The listing builds one solid part. Answer for the finished solid, in the listing's coordinates (mm). Give positions to 0.01 mm unless a question says otherwise; leave off trailing zeros. Write each loop counter-clockwise with the first axis right and the second up, starting at its lowest first coordinate (ties: lowest second). Pieces come first, ordered by that corner, then holes. Notation, with made-up numbers: (43.5, 58.25) - (74.5, 58.25) arc R20 cw to (74.5, 90.25) - close; hole circle Ø1 at (-12, 5.25). An arc over 180 degrees is marked (long way). Answer as CSV lines item,"result". Start each with the question number.
(1) Find section A-A (y = 77.5). Write down the section's boundary in (x, z), then the cut area to 4 significant figures.
(2) Find section D-D (y = 56.5). Write down the section's boundary in (x, z), then the cut area to 3 significant figures.
(3) Straight lines are drawn through the part: probe 1 along Y at (x, z) = (21.25, 6.75); probe 2 along Y at (x, z) = (16.5, 0.5); probe 3 along X at (y, z) = (34, 0.75). For each, find the intervals that lie inside material, in ascending order.
(4) Each of these flat-tipped pins is pushed along its axis until it touches: pin 1 Ø1.5 at (x, z) = (29.5, 6.5) entering from +Y; pin 2 Ø5 at (y, z) = (29, 8.5) entering from -X; pin 3 Ø7.5 at (x, y) = (21.25, 77.5) entering from -Z; pin 4 Ø5 at (x, z) = (124.5, 4.5) entering from +Y. Where does it stop, or does it pass through?
(5) For a pull along Y with two mould halves and no side action, classify faces 1 (the face through (20.436, 83.697, 4.93)), 2 (the face through (82, -1.25, 5)), 3 (the face through (74, 49, 0)) as pulls with the +Y half, pulls with the -Y half, needs draft (parallel to the pull), parting line crosses it, or undercut.
(6) Find section B-B (z = 2.25). Write down the section's boundary in (x, y), then the cut area to 3 significant figures.
(7) Find section C-C (x = 22). Write down the section's boundary in (y, z).
from build123d import *

# Parameters (mm, degrees)
F0_R        = 6.25
F1_DEPTH    = 10
F2_T1_DEPTH = 18.1439634323
F2_T3_DEPTH = 61.4336597593
F3_R        = 10


# Not quite as in the source:
# - a fillet or chamfer that OpenCascade refuses, or shapes differently, is made with other operations: its cross-section is extruded or revolved along the edge and cut away or added
# - two fillets or chamfers of one size are made in one step


with BuildPart() as f1:
    # F0 (on Top) → F1 (new body)
    with BuildSketch(Plane.XY):
        Polygon((0, 73.75), (15, -1.25), (150, -1.25), (150, 68.75), (30, 98.75), (0, 98.75), align=None)
        with Locations((21.25, 77.5)):
            Circle(F0_R, mode=Mode.SUBTRACT)
    extrude(amount=F1_DEPTH)

    # F2: chamfer of 10 on 2 edges, made by hand

    # F2_s2 → F2_t1 (cut)
    with BuildSketch(Plane.XY.offset(-4.0719817161)):
        Polygon((31.1942999942, 98.4514250015), (28.7689437438, 98.75), (30, 98.75), align=None)
    extrude(amount=F2_T1_DEPTH, mode=Mode.SUBTRACT)

    # F2_s4 → F2_t3 (cut)
    with BuildSketch(Plane.XY.offset(-25.7168298797)):
        Polygon((10, 98.75), (0, 88.75), (0, 98.75), align=None)
    extrude(amount=F2_T3_DEPTH, mode=Mode.SUBTRACT)

    # F3
    f3_edges = [f1.edges().sort_by_distance(p)[0] for p in [
        (0, 88.75, 5),
        (10, 98.75, 5),
        (28.768944, 98.75, 5),
    ]]
    fillet(f3_edges, radius=F3_R)


solid = f1.part
Result set:
1,outline,"(0, 0) - (15, 0) - (15, 10) - (0, 10) - close; (27.5, 0) - (115, 0) - (115, 10) - (27.5, 10) - close"
1,area,"1,025 mm^2"
2,outline,"(3.45, 0) - (150, 0) - (150, 10) - (3.45, 10) - close"
2,area,"1,470 mm^2"
3,probe 1,"-1.25 to 71.25, 83.75 to 98.75"
3,probe 2,"-1.25 to 73.44, 81.56 to 98.75"
3,probe 3,"7.95 to 150"
4,pin 1,"y = 98.73"
4,pin 2,"x = 8.45"
4,pin 3,"through"
4,pin 4,"y = 75.75"
5,face 1,"undercut"
5,face 2,"pulls with the -Y half"
5,face 3,"needs draft"
6,outline,"(0, 73.75) - (15, -1.25) - (150, -1.25) - (150, 68.75) - (31.19, 98.45) - (29.38, 98.68) arc R10 ccw to (28.16, 98.75) - (14.14, 98.75) arc R10 ccw to (7.07, 95.82) - (2.93, 91.68) arc R10 ccw to (0, 84.61) - close; hole circle Ø12.5 at (21.25, 77.5)"
6,area,"12,500 mm^2"
7,outline,"(-1.25, 0) - (71.3, 0) - (71.3, 10) - (-1.25, 10) - close; (83.7, 0) - (98.75, 0) - (98.75, 10) - (83.7, 10) - close"
